Geometry check sheet. Reference: the model listing, model coordinates, mm. Face numbers are marked on the shaded views. Round coordinates to 2 decimals unless told otherwise and drop trailing zeros. Loops run counter-clockwise (first coordinate to the right, second up) from the corner with the lowest first, then second, coordinate; pieces in that order, holes last. Notation, with made-up numbers: M 29,-21 L 62,-21 A28 ccw 62,5 Z; hole C 74.25,16.5 d2. An arc over 180 degrees is marked long. Write item = value, one per line.
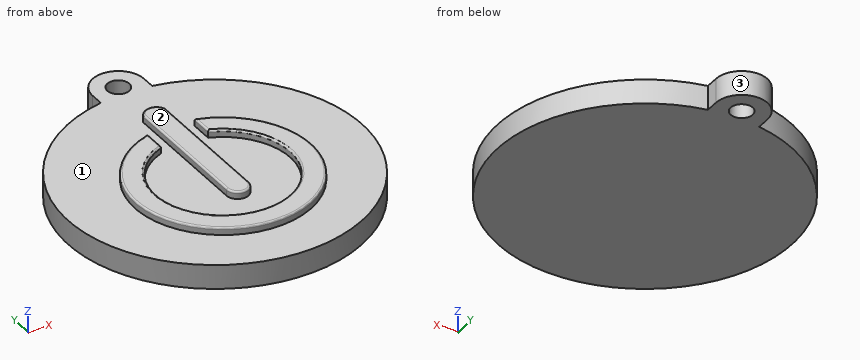
from build123d import *

# Parameters (mm, degrees)
EXTRUDE_DEPTH = 3.3
SKETCH001_R   = 1.5
POCKET_DEPTH  = 3.301
PAD_DEPTH     = 1
FILLET_R      = 0.25


with BuildPart() as part:
    # Sketch → Extrude (new body)
    with BuildSketch(Plane.XY):
        with BuildLine():
            ThreePointArc((3.5, 21.5), (0, 25), (-3.5, 21.5))
            Line((-3.5, 21.5), (-3.5, 19.691369))
            ThreePointArc((-3.5, 19.691369), (0, -20), (3.5, 19.691369))
            Line((3.5, 19.691369), (3.5, 21.5))
        make_face()
    extrude(amount=EXTRUDE_DEPTH)

    # Sketch001 (on Face6 of Extrude) → Pocket (cut, through all)
    with BuildSketch(Plane.XY.offset(3.3)):
        with Locations((0, 21.5)):
            Circle(SKETCH001_R)
    extrude(amount=-POCKET_DEPTH, mode=Mode.SUBTRACT)

    # Sketch002 (on Face1 of CopyClone) → Pad (join)
    with BuildSketch(Plane.XY.offset(3.3)):
        with BuildLine():
            Line((-1.5, 13.5), (-1.5, -5))
            ThreePointArc((-1.5, -5), (0, -6.5), (1.5, -5))
            Line((1.5, 13.5), (1.5, -5))
            ThreePointArc((1.5, 13.5), (0, 14.581139), (-1.5, 13.5))
        make_face()
        with BuildLine():
            Line((-3.2, 9.765466), (-3.2, 6.765466))
            ThreePointArc((-3.2, 6.765466), (0, -10.943698), (3.2, 6.765466))
            Line((3.2, 9.765466), (3.2, 6.765466))
            ThreePointArc((-3.2, 9.765466), (0, -13.8), (3.2, 9.765466))
        make_face()
    extrude(amount=PAD_DEPTH)

    # Fillet
    fillet_edges = [part.edges().sort_by_distance(p)[0] for p in [
        (0, 14.581139, 4.3),
        (1.5, 4.25, 4.3),
        (0, -6.5, 4.3),
        (-1.5, 4.25, 4.3),
        (-3.2, 8.265466, 4.3),
        (0, -10.943698, 4.3),
        (3.2, 8.265466, 4.3),
        (0, -13.8, 4.3),
    ]]
    fillet(fillet_edges, radius=FILLET_R)


solid = part.part
(1) Material ranges on line 1 along X through (y, z) = (-1.8, 3.5); line 2 along Y through (x, z) = (0, 1.8); line 3 along Z through (x, y) = (-9, -10), recorded low to high. Write a range as from..to.
Result set:
line_1 = -12..-9.14, -1.5..1.5, 9.14..12
line_2 = -20..20, 23..25
line_3 = 0..3.3
(2) Release check for a two-part mould opening along X. For the marked faces 1, 2 and 3 record: released by +X, released by -X, zero draft, split by the parting line, or undercut.
Result set:
face_1 = undercut
face_2 = zero draft
face_3 = split by the parting line
(3) Sectioned sample at B-B on z = 0.8. Record the cut outline in (x, y).
Result set:
outline = M -3.5,19.69 A20 ccw long 3.5,19.69 L 3.5,21.5 A3.5 ccw -3.5,21.5 Z; hole C 0,21.5 d3
(4) Sectioned sample at D-D on x = -14. Record the cut outline in (y, z).
Result set:
outline = M -14.28,0 L 14.28,0 L 14.28,3.3 L -14.28,3.3 Z
(5) Sectioned sample at A-A on x = 0. Record the cut outline in (y, z).
Result set:
outline = M -20,0 L 20,0 L 20,3.3 L 14.58,3.3 L 14.58,4.05 A0.25 ccw 14.33,4.3 L -6.25,4.3 A0.25 ccw -6.5,4.05 L -6.5,3.3 L -10.94,3.3 L -10.94,4.05 A0.25 ccw -11.19,4.3 L -13.55,4.3 A0.25 ccw -13.8,4.05 L -13.8,3.3 L -20,3.3 Z; M 23,0 L 25,0 L 25,3.3 L 23,3.3 Z
(6) Depth check by flat-ended pin: pin 1 Ø2 at (x, z) = (-2.5, 0.5) entering from -Y; pin 2 Ø1.4 at (y, z) = (21, 2.5) entering from -X; pin 3 Ø0.6 at (y, z) = (8.5, 3.5) entering from +X. Enter the tip coordinate at first touch or a pass-through.
Result set:
pin_1 = -19.94
pin_2 = -3.5
pin_3 = 18.21
(7) Sectioned sample at C-C on y = -16.5. Record the cut outline in (x, z).
Result set:
outline = M -11.3,0 L 11.3,0 L 11.3,3.3 L -11.3,3.3 Z
